Answer from the drawing. Dimensions are ordinates in mm from the lowest x, y and z of the part. A direction names the side the tool comes from. Round coordinates to 2 decimals unless told otherwise and drop trailing zeros. Order: outer loops, then holes, each group sorted by start corner. A loop starts at its lowest first (then second) coordinate and runs counter-clockwise, first axis right, second up. Notation, with made-up numbers: (-33.75, -8) -> (25.25, -8) arc R15 ccw to (25.25, 19) -> close; hole circle Ø10 at (14.5, 80.5). An arc over 180 degrees is marked (long way). Use a Markdown table: item, result. Add a question column.
1. The mould has two halves that part along Y. Classify the marked faces 1, 2 and 3: +Y half, -Y half, draft (parallel to the pull), parting line (faces both ways), or undercut.
2. Given pin 1 (10 mm diameter, centred on y = 22.5, z = 20.5, fed in from +X); pin 2 (3 mm diameter, centred on x = 17, y = 34, fed in from +Z); pin 3 (2 mm diameter, centred on y = 46, z = 39.5, fed in from +X), each flat-ended and moving along its own axis, determine where each tip first touches the part or whether it passes through.
3. Consider L1, parallel to Y at x = 6.5, z = 40.5 (3 decimals); L2, parallel to Z at x = 25, y = 25; L3, parallel to Y at x = 16, z = 32.5. Determine where each line is inside the solid, lowest interval first. Write a range as [from, to].
4. For the marked faces 4 and 5, determine the directions among +Z, -Z, +X, -X, +Y, -Y from which every point of the face is accessible in a straight line to the end or side of a thin tool.
5. Section D-D, the plane x = 17.5 is taken. Give the vertices of the cut face in (y, z) (1 decimal).
6. Section B-B, the plane x = 25 is taken. Give the vertices of the cut face in (y, z) (3 decimals), then the cut area to 3 significant figures.
7. Section C-C, the plane y = 47.5 is taken. Give the vertices of the cut face in (x, z).
8. Section A-A, the plane z = 25 is taken. Give the vertices of the cut face in (x, y) (3 decimals).
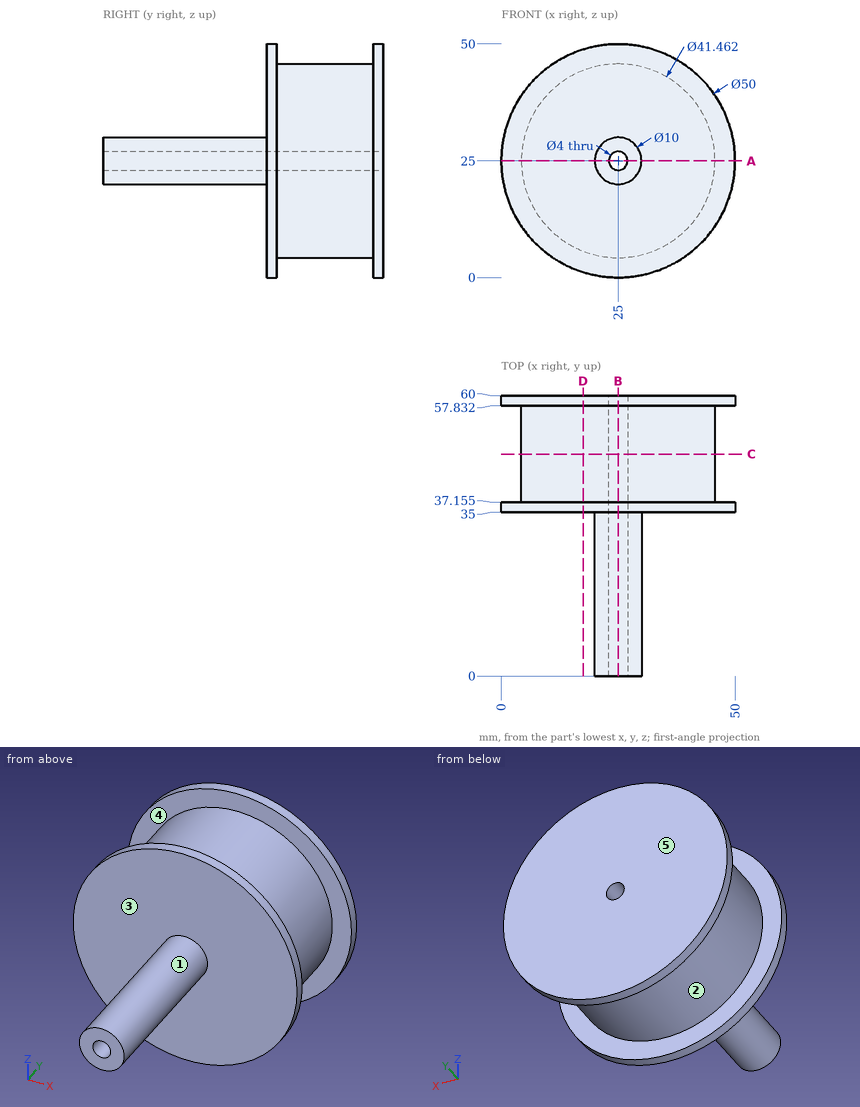
Verdict:
| question | item | result |
|---|---|---|
| 1 | face 1 | draft |
| 1 | face 2 | undercut |
| 1 | face 3 | -Y half |
| 2 | pin 1 | stops at x = 30 |
| 2 | pin 2 | stops at z = 49.03 |
| 2 | pin 3 | stops at x = 40.73 |
| 3 | L1 | y = [35, 37.155], [57.832, 60] |
| 3 | L2 | z = [20, 23], [27, 30] |
| 3 | L3 | y = [35, 60] |
| 4 | face 4 | none |
| 4 | face 5 | +Z, -Z, +X, -X, +Y |
| 5 | outline | (35, 1.2) -> (37.2, 1.2) -> (37.2, 5.7) -> (57.8, 5.7) -> (57.8, 1.2) -> (60, 1.2) -> (60, 48.8) -> (57.8, 48.8) -> (57.8, 44.3) -> (37.2, 44.3) -> (37.2, 48.8) -> (35, 48.8) -> close |
| 6 | outline | (0, 20) -> (35, 20) -> (35, 0) -> (37.155, 0) -> (37.155, 4.269) -> (57.832, 4.269) -> (57.832, 0) -> (60, 0) -> (60, 23) -> (0, 23) -> close; (0, 27) -> (60, 27) -> (60, 50) -> (57.832, 50) -> (57.832, 45.731) -> (37.155, 45.731) -> (37.155, 50) -> (35, 50) -> (35, 30) -> (0, 30) -> close |
| 6 | area | 1,180 mm2 |
| 7 | outline | circle Ø41.46 at (25, 25); hole circle Ø4 at (25, 25) |
| 8 | outline | (0, 35) -> (20, 35) -> (20, 0) -> (23, 0) -> (23, 60) -> (0, 60) -> (0, 57.832) -> (4.269, 57.832) -> (4.269, 37.155) -> (0, 37.155) -> close; (27, 0) -> (30, 0) -> (30, 35) -> (50, 35) -> (50, 37.155) -> (45.731, 37.155) -> (45.731, 57.832) -> (50, 57.832) -> (50, 60) -> (27, 60) -> close |
